```python
from build123d import *

# Parameters (mm, degrees)
F1_ANGLE  = 180
F3_DEPTH  = 5
F5_DEPTH  = 5
F7_DEPTH  = 3
F9_DEPTH  = 17
F11_DEPTH = 17
F13_DEPTH = 3
F15_DEPTH = 17
F17_DEPTH = 17
F19_DEPTH = 3
F21_DEPTH = 3
F22_W     = 11.3347762211
F22_H     = 1.4
F23_DEPTH = 4
F24_W     = 11.3347762211
F24_H     = 2.4
F25_DEPTH = 5
F27_DEPTH = 11.3347762211
F28_W     = 11.3347762211
F28_H     = 5
F29_DEPTH = 1
F31_DEPTH = 11.3347762211
F32_W     = 11.3347762211
F32_H     = 5
F33_DEPTH = 1
F35_DEPTH = 11.3347762211
F37_DEPTH = 11.3347762211


with BuildPart() as f1:
    # F0 (on Top) → F1 (revolve)
    with BuildSketch(Plane.XY):
        with BuildLine():
            ThreePointArc((-75, 7), (0, 12), (75, 7))
            Line((75, 7), (92, 7))
            Line((92, 7), (92, 10))
            Line((92, 10), (75, 10))
            ThreePointArc((75, 10), (0, 15), (-75, 10))
            Line((-75, 10), (-92, 10))
            Line((-92, 10), (-92, 7))
            Line((-92, 7), (-75, 7))
        make_face()
    revolve(axis=Axis((-37.5, 0, 0), (-1, 0, 0)), revolution_arc=F1_ANGLE)

    # F2 (on face) → F3 (join)
    with BuildSketch(Plane.XY):
        with BuildLine():
            Line((-75, 10), (-92, 10))
            Line((-92, 10), (-92, 7))
            Line((-92, 7), (-75, 7))
            ThreePointArc((-75, 7), (0, 12), (75, 7))
            Line((75, 7), (92, 7))
            Line((92, 7), (92, 10))
            Line((92, 10), (75, 10))
            ThreePointArc((75, 10), (0, 15), (-75, 10))
        make_face()
        with BuildLine():
            Line((-75.4652237789, 17), (-92, 17))
            Line((-92, 17), (-92, 10))
            Line((-92, 10), (-75, 10))
            ThreePointArc((-75, 10), (0, 15), (75, 10))
            Line((75, 10), (92, 10))
            Line((92, 10), (92, 17))
            Line((92, 17), (75.4652237789, 17))
            ThreePointArc((75.4652237789, 17), (0, 22), (-75.4652237789, 17))
        make_face()
    extrude(amount=-F3_DEPTH)

    # F4 (on face) → F5 (join)
    with BuildSketch(Plane.XY):
        with BuildLine():
            Line((-92, -7), (-92, -10))
            Line((-92, -10), (-75, -10))
            ThreePointArc((-75, -10), (0, -15), (75, -10))
            Line((75, -10), (92, -10))
            Line((92, -10), (92, -7))
            Line((92, -7), (75, -7))
            ThreePointArc((75, -7), (0, -12), (-75, -7))
            Line((-75, -7), (-92, -7))
        make_face()
        with BuildLine():
            Line((-92, -10), (-92, -17))
            Line((-92, -17), (-75.4652237789, -17))
            ThreePointArc((-75.4652237789, -17), (0, -22), (75.4652237789, -17))
            Line((75.4652237789, -17), (92, -17))
            Line((92, -17), (92, -10))
            Line((92, -10), (75, -10))
            ThreePointArc((75, -10), (0, -15), (-75, -10))
            Line((-75, -10), (-92, -10))
        make_face()
    extrude(amount=-F5_DEPTH)

    # F6 (on face) → F7 (cut)
    with BuildSketch(Plane.XY):
        with BuildLine():
            Line((-75.3060422543, 14.6), (-92, 14.6))
            Line((-92, 14.6), (-92, 7))
            Line((-92, 7), (-75, 7))
            Line((-75, 7), (-75, 8.8160197075))
            ThreePointArc((-75, 8.8160197075), (0, 13.8), (75, 8.8160197075))
            Line((75, 8.8160197075), (75, 7))
            Line((75, 7), (92, 7))
            Line((92, 7), (92, 14.6))
            Line((92, 14.6), (75.3060422543, 14.6))
            ThreePointArc((75.3060422543, 14.6), (0, 19.6), (-75.3060422543, 14.6))
        make_face()
        with BuildLine():
            Line((-75, 8.8160197075), (-75, 7))
            ThreePointArc((-75, 7), (0, 12), (75, 7))
            Line((75, 7), (75, 8.8160197075))
            ThreePointArc((75, 8.8160197075), (0, 13.8), (-75, 8.8160197075))
        make_face()
    extrude(amount=-F7_DEPTH, mode=Mode.SUBTRACT)

    # F8 (on face) → F9 (cut)
    with BuildSketch(Plane(origin=(-92, 0, 0), x_dir=(0, -1, 0), z_dir=(-1, 0, 0))):
        with BuildLine():
            Line((-7, 0), (-7, -3))
            Line((-7, -3), (-6.3245553203, -3))
            ThreePointArc((-6.3245553203, -3), (-6.8290514437, -1.5375488216), (-7, 0))
        make_face()
    extrude(amount=-F9_DEPTH, mode=Mode.SUBTRACT)

    # F10 (on face) → F11 (cut)
    with BuildSketch(Plane.YZ.offset(92)):
        with BuildLine():
            Line((6.3245553203, -3), (7, -3))
            Line((7, -3), (7, 0))
            ThreePointArc((7, 0), (6.8290514437, -1.5375488216), (6.3245553203, -3))
        make_face()
    extrude(amount=-F11_DEPTH, mode=Mode.SUBTRACT)

    # F12 (on face) → F13 (cut)
    with BuildSketch(Plane.XY):
        with BuildLine():
            Line((-92, -7), (-92, -8.8))
            Line((-92, -8.8), (-75.1199041533, -8.8))
            ThreePointArc((-75.1199041533, -8.8), (-75.059952504, -8.8080130526), (-75, -8.8160197075))
            Line((-75, -8.8160197075), (-75, -7))
            Line((-75, -7), (-92, -7))
        make_face()
        with BuildLine():
            Line((-92, -8.8), (-92, -14.6))
            Line((-92, -14.6), (-75.3060422543, -14.6))
            ThreePointArc((-75.3060422543, -14.6), (0, -19.6), (75.3060422543, -14.6))
            Line((75.3060422543, -14.6), (92, -14.6))
            Line((92, -14.6), (92, -8.8))
            Line((92, -8.8), (75.1199041533, -8.8))
            ThreePointArc((75.1199041533, -8.8), (75.059952504, -8.8080130526), (75, -8.8160197075))
            ThreePointArc((75, -8.8160197075), (0, -13.8), (-75, -8.8160197075))
            ThreePointArc((-75, -8.8160197075), (-75.059952504, -8.8080130526), (-75.1199041533, -8.8))
            Line((-75.1199041533, -8.8), (-92, -8.8))
        make_face()
        with BuildLine():
            Line((75.1199041533, -8.8), (92, -8.8))
            Line((92, -8.8), (92, -7))
            Line((92, -7), (75, -7))
            Line((75, -7), (75, -8.8160197075))
            ThreePointArc((75, -8.8160197075), (75.059952504, -8.8080130526), (75.1199041533, -8.8))
        make_face()
    extrude(amount=-F13_DEPTH, mode=Mode.SUBTRACT)

    # F14 (on face) → F15 (cut)
    with BuildSketch(Plane(origin=(-92, 0, 0), x_dir=(0, -1, 0), z_dir=(-1, 0, 0))):
        with BuildLine():
            Line((6.3245553203, -3), (7, -3))
            Line((7, -3), (7, 0))
            ThreePointArc((7, 0), (6.8290514437, -1.5375488216), (6.3245553203, -3))
        make_face()
    extrude(amount=-F15_DEPTH, mode=Mode.SUBTRACT)

    # F16 (on face) → F17 (cut)
    with BuildSketch(Plane.YZ.offset(92)):
        with BuildLine():
            Line((-7, 0), (-7, -3))
            Line((-7, -3), (-6.3245553203, -3))
            ThreePointArc((-6.3245553203, -3), (-6.8290514437, -1.5375488216), (-7, 0))
        make_face()
    extrude(amount=-F17_DEPTH, mode=Mode.SUBTRACT)

    # F18 (on face) → F19 (cut)
    with BuildSketch(Plane.XY):
        with BuildLine():
            ThreePointArc((75, 7), (0, 12), (-75, 7))
            Line((-75, 7), (-75, 5.4070060141))
            Line((-75, 5.4070060141), (75, 5.4070060141))
            Line((75, 5.4070060141), (75, 7))
        make_face()
    extrude(amount=-F19_DEPTH, mode=Mode.SUBTRACT)

    # F20 (on face) → F21 (cut)
    with BuildSketch(Plane.XY):
        with BuildLine():
            Line((-75, -5.2931243554), (-75, -7))
            ThreePointArc((-75, -7), (0, -12), (75, -7))
            Line((75, -7), (75, -5.2931243554))
            Line((75, -5.2931243554), (-75, -5.2931243554))
        make_face()
        with BuildLine():
            Line((-75, -7), (-75, -8.8160197075))
            ThreePointArc((-75, -8.8160197075), (0, -13.8), (75, -8.8160197075))
            Line((75, -8.8160197075), (75, -7))
            ThreePointArc((75, -7), (0, -12), (-75, -7))
        make_face()
    extrude(amount=-F21_DEPTH, mode=Mode.SUBTRACT)

    # F22 (on face) → F23 (join)
    with BuildSketch(Plane.XY):
        with Locations((83.7326118895, 15.3)):
            Rectangle(F22_W, F22_H)
        with Locations((-83.7326118895, 15.3)):
            Rectangle(F22_W, F22_H)
    extrude(amount=F23_DEPTH)

    # F24 (on face) → F25 (join)
    with BuildSketch(Plane.XY):
        with Locations((83.7326118895, -15.8)):
            Rectangle(F24_W, F24_H)
        with Locations((-83.7326118895, -15.8)):
            Rectangle(F24_W, F24_H)
    extrude(amount=F25_DEPTH)

    # F26 (on face) → F27 (join, through all)
    with BuildSketch(Plane(origin=(-89.4, 0, 0), x_dir=(0, -1, 0), z_dir=(-1, 0, 0))):
        Polygon((13.1, 3.2), (13.1, 2), (14.6, 2), (14.6, 5), align=None)
    extrude(amount=-F27_DEPTH)

    # F28 (on face) → F29 (cut)
    with BuildSketch(Plane.XZ.offset(17)):
        with Locations((-83.7326118895, 2.5)):
            Rectangle(F28_W, F28_H)
    extrude(amount=-F29_DEPTH, mode=Mode.SUBTRACT)

    # F30 (on face) → F31 (join, through all)
    with BuildSketch(Plane.YZ.offset(89.4)):
        Polygon((-14.6, 5), (-14.6, 2), (-13.1, 2), (-13.1, 3.2), align=None)
    extrude(amount=-F31_DEPTH)

    # F32 (on face) → F33 (cut)
    with BuildSketch(Plane.XZ.offset(17)):
        with Locations((83.7326118895, 2.5)):
            Rectangle(F32_W, F32_H)
    extrude(amount=-F33_DEPTH, mode=Mode.SUBTRACT)

    # F34 (on face) → F35 (join, through all)
    with BuildSketch(Plane.YZ.offset(89.4)):
        Polygon((13.1, 1), (14.6, 1), (14.6, 4), (13.1, 2.2), align=None)
    extrude(amount=-F35_DEPTH)

    # F36 (on face) → F37 (join, through all)
    with BuildSketch(Plane(origin=(-89.4, 0, 0), x_dir=(0, -1, 0), z_dir=(-1, 0, 0))):
        Polygon((-14.6, 4), (-14.6, 1), (-13.1, 1), (-13.1, 2.2), align=None)
    extrude(amount=-F37_DEPTH)


solid = f1.part
```
Part model, mm, in its own coordinate system. A direction names the side the tool comes from. Round coordinates to 2 decimals unless told otherwise and drop trailing zeros. Use one line per item in the form item = value. Start each with the question number.
Item 1: Two-plate mould, pull along Z, no slides. Class faces 6 (the flat face through (84, -17, -2)), 7 (the flat face through (84, 14.6, -1)), 8 (the flat face through (-1, 15, -5)): released by +Z, released by -Z, zero draft, split by the parting line, or undercut.
Item 2: Drill centre lines: line 1 along Y through (x, z) = (-25, -13); line 2 along Y through (x, z) = (0.5, -8); line 3 along Z through (x, y) = (-82.5, -14). Where is each one in solid material? Low to high.
Item 3: Drop flat-ended pins along their axis: pin 1 Ø1.1 at (x, y) = (82.5, 15) entering from +Z; pin 2 Ø2 at (x, y) = (4, -18.5) entering from +Z; pin 3 Ø0.8 at (x, y) = (81, 14) entering from -Z. Give the stop position or say it passes through.
Item 4: Tool access for faces 1 (the flat face through (84, 16, 2)), 2 (the flat face through (-89.4, -15, 3)), 3 (the cylindrical face through (1.1, 19.6, -1.5)), 4 (the flat face through (84, -14.6, 0)), 5 (the flat face through (-78.065, 15, 2)): list every direction of +Z, -Z, +X, -X, +Y, -Y with a clear straight run to the whole face (end or side of a thin tool).
Data:
q1.face_6 = zero draft
q1.face_7 = undercut
q1.face_8 = released by -Z
q2.line_1 = -6.3 to 6.3
q2.line_2 = -12.69 to -8.94, 8.94 to 12.69
q2.line_3 = -5 to -3, 2 to 4.28
q3.pin_1 = 4
q3.pin_2 = -3
q3.pin_3 = -5
q4.face_1 = +Z, +X, -X, +Y
q4.face_2 = +Z, -X, +Y, -Y
q4.face_3 = +Z
q4.face_4 = +X, -X
q4.face_5 = +Z, +Y, -Y
